The model under review builds one solid part; all positions refer to its coordinate system, in mm. Coordinates: 2 decimals unless noted, no trailing zeros. Loops run counter-clockwise (first coordinate to the right, second up) from the corner with the lowest first, then second, coordinate; pieces in that order, holes last. Notation, with made-up numbers: M 58.25,13.25 L 85.25,13.25 A22 cw 85.25,26.25 Z; hole C 59.5,-11.75 d2. An arc over 180 degrees is marked long. Use CSV: the item, a comma, the result in double quotes. Start each with the question number.
1. Clearance check with flat-ended pins moving along their axes: P1, Ø1.2, axis at x = -0.5, y = 0.5, coming from the -Z side; P2, Ø1.5, axis at y = 0, z = -5, coming from the -X side. State where each tip first meets the part, or that it passes through.
2. Add section D-D, the plane y = 1.6. Write out the cut boundary in (x, z), then the cut area to 3 significant figures.
3. For L1, parallel to Y at x = 0, z = 0.8 (3 decimals); L2, parallel to Z at x = -1.1, y = -0.8; L3, parallel to X at y = 0.9, z = -4 (3 decimals), list the stretches that pass through material, from the lowest coordinate up.
4. Add section C-C, the plane z = -0.5. Write out the cut boundary in (x, y) (3 decimals).
5. Add section A-A, the plane y = 0. Write out the cut boundary in (x, z) (3 decimals), then the cut area to 3 significant figures.
6. Draft analysis for pull direction Y (two halves, no side actions). For faces 1 (the flat face through (-1, 1, 0)), 2 (the cylindrical face through (-0.37, -1.66, 0.88)), 3 (the cylindrical face through (-1.57, -1.2, 0.74)), state which applies: +Y half, -Y half, draft (parallel to the pull), parting line (faces both ways), or undercut.
from build123d import *

# Parameters (mm, degrees)
ESQUISSE1_R             = 1.975
BOSS_EXTRU_1_DEPTH      = 1.5
ESQUISSE2_R             = 1.25
BOSS_EXTRU_2_DEPTH      = 6
ESQUISSE3_R             = 1.7
ENL_V_MAT_EXTRU_2_DEPTH = 1.25
ESQUISSE4_R             = 1.125
ENL_V_MAT_EXTRU_4_DEPTH = 51.25


with BuildPart() as part:
    # Esquisse1 → Boss.-Extru.1 (new body)
    with BuildSketch(Plane.XY):
        Circle(ESQUISSE1_R)
    extrude(amount=BOSS_EXTRU_1_DEPTH)

    # Esquisse2 → Boss.-Extru.2 (add)
    with BuildSketch(Plane(origin=(0, 0, 0), x_dir=(-1, 0, 0), z_dir=(0, 0, -1))):
        Circle(ESQUISSE2_R)
    extrude(amount=BOSS_EXTRU_2_DEPTH)

    # Esquisse3 → Enlèv. mat.-Extru.2 (cut)
    with BuildSketch(Plane.XY.offset(1.5)):
        Circle(ESQUISSE3_R)
    extrude(amount=-ENL_V_MAT_EXTRU_2_DEPTH, mode=Mode.SUBTRACT)

    # Esquisse4 → Enlèv. mat.-Extru.4 (cut)
    with BuildSketch(Plane(origin=(0, 0, -6), x_dir=(-1, 0, 0), z_dir=(0, 0, -1))):
        Circle(ESQUISSE4_R)
    extrude(amount=-ENL_V_MAT_EXTRU_4_DEPTH, mode=Mode.SUBTRACT)


solid = part.part
Computed:
1,P1,"stops at z = -6"
1,P2,"stops at x = -1.25"
2,outline,"M -1.16,0 L 1.16,0 L 1.16,1.5 L 0.57,1.5 L 0.57,0.25 L -0.57,0.25 L -0.57,1.5 L -1.16,1.5 Z"
2,area,"2.04 mm^2"
3,L1,"y = -1.975 to -1.7, 1.7 to 1.975"
3,L2,"z = 0 to 0.25"
3,L3,"x = -0.867 to -0.675, 0.675 to 0.867"
4,outline,"C 0,0 d2.5; hole C 0,0 d2.25"
5,outline,"M -1.975,0 L -1.25,0 L -1.25,-6 L -1.125,-6 L -1.125,0.25 L -1.7,0.25 L -1.7,1.5 L -1.975,1.5 Z; M 1.125,-6 L 1.25,-6 L 1.25,0 L 1.975,0 L 1.975,1.5 L 1.7,1.5 L 1.7,0.25 L 1.125,0.25 Z"
5,area,"2.61 mm^2"
6,face 1,"draft"
6,face 2,"undercut"
6,face 3,"parting line"
